The model under review builds one solid part; all positions refer to its coordinate system, in mm. A direction names the side the tool comes from. Give positions to 0.01 mm unless a question says otherwise; leave off trailing zeros. Write each loop counter-clockwise with the first axis right and the second up, starting at its lowest first coordinate (ties: lowest second). Pieces come first, ordered by that corner, then holes. Notation, with made-up numbers: M 6.25,-4.75 L 39.25,-4.75 A26 ccw 39.25,9.25 Z; hole C 43,-4 d5. An arc over 180 degrees is marked long. Write each question's results on one line, items separated by ' | '. Start each with the question number.
Autodesk Inventor part; units mm, degrees
ref_plane "YZ Plane" through (0, 0, 0) normal (1, 0, 0) x (0, 1, 0)
ref_plane "XZ Plane" through (0, 0, 0) normal (0, 1, 0) x (-1, 0, 0)
ref_plane "XY Plane" through (0, 0, 0) normal (0, 0, 1) x (1, 0, 0)
sketch "Sketch1" plane through (0, 0, 0) normal (0, 1, 0) x (-1, 0, 0)
  line L0 (17.75, -20.2435) -> (17.75, -42.6397) construction
  line L1 (13.2323, -33.7) -> (6.4845, -33.7) construction
  line L2 (35.5, -64.4) -> (35.5, -3)
  line L3 (0, -3) -> (0, -64.4)
  line L4 (32.5, 0) -> (3, 0)
  line L5 (3, -67.4) -> (32.5, -67.4)
  line L6 (16, -20.2) -> (14.2, -20.2)
  line L7 (14.2, -20.2) -> (14.2, -13.2)
  line L8 (14.2, -13.2) -> (16, -13.2)
  line L9 (16, -13.2) -> (16, -20.2)
  line L10 (31.25, -3) -> (21.25, -3)
  line L11 (21.25, -3) -> (21.25, -6.2)
  line L12 (21.25, -6.2) -> (31.25, -6.2)
  line L13 (31.25, -6.2) -> (31.25, -3)
  line L14 (14.25, -3) -> (4.25, -3)
  line L15 (4.25, -3) -> (4.25, -6.2)
  line L16 (4.25, -6.2) -> (14.25, -6.2)
  line L17 (14.25, -6.2) -> (14.25, -3)
  line L18 (31.25, -61.2) -> (21.25, -61.2)
  line L19 (21.25, -61.2) -> (21.25, -64.4)
  line L20 (21.25, -64.4) -> (31.25, -64.4)
  line L21 (31.25, -64.4) -> (31.25, -61.2)
  line L22 (14.25, -61.2) -> (4.25, -61.2)
  line L23 (4.25, -61.2) -> (4.25, -64.4)
  line L24 (4.25, -64.4) -> (14.25, -64.4)
  line L25 (14.25, -64.4) -> (14.25, -61.2)
  line L26 (10.7, -28.7) -> (7.5, -28.7)
  line L27 (7.5, -28.7) -> (7.5, -38.7)
  line L28 (7.5, -38.7) -> (10.7, -38.7)
  line L29 (10.7, -28.7) -> (10.7, -26.2)
  line L30 (10.7, -26.2) -> (13.9, -26.2)
  line L31 (13.9, -26.2) -> (13.9, -41.2)
  line L32 (13.9, -41.2) -> (10.7, -41.2)
  line L33 (10.7, -41.2) -> (10.7, -38.7)
  arc A0 (35.5, -3) -> (32.5, 0) centre (32.5, -3) ccw
  arc A1 (32.5, -67.4) -> (35.5, -64.4) centre (32.5, -64.4) ccw
  arc A2 (0, -64.4) -> (3, -67.4) centre (3, -64.4) ccw
  arc A3 (3, 0) -> (0, -3) centre (3, -3) ccw
  line L34 (16, -47.2) -> (14.2, -47.2)
  line L35 (14.2, -47.2) -> (14.2, -54.2)
  line L36 (14.2, -54.2) -> (16, -54.2)
  line L37 (16, -54.2) -> (16, -47.2)
  point P0 (0, 0)
  dimension "d22" = 7
  dimension "d24" = 1.8
  dimension "d27" = 10
  dimension "d28" = 3.2
  dimension "d30" = 3
  dimension "d31" = 7
  dimension "d33" = 10
  dimension "d34" = 15
  dimension "d35" = 6
  dimension "d39" = 7
  dimension "d52" = 35.5
  dimension "d53" = 4.25
  dimension "d54" = 7.5
  dimension "d55" = 3.5
  dimension "d56" = 55
extrude "Extrusion1" add sketch "Sketch1" along normal blind 3
properties part number "Front_wall"
(1) Add section B-B (x = -9). State the section outline as (y, z) points.
(2) Draft analysis for pull direction Z (two halves, no side actions). For faces 1 (the flat face through (-18, 3, -33)), 2 (the flat face through (-14.25, 1, -5)), 3 (the cylindrical face through (-0.9, 1.48, -66.54)), state which applies: pulls with the +Z half, pulls with the -Z half, needs draft (parallel to the pull), parting line crosses it, or undercut.
(3) Machinability: for faces 4 (the flat face through (-9, 1, -38.7)), 5 (the cylindrical face through (-34.64, 1.48, -66.5)), which of the approach directions +Z, -Z, +X, -X, +Y, -Y give a long, thin tool a straight path to every point of the face, cutting with its end or side? Answer none if there is none.
(4) Wall thickness on L1, parallel to Z at x = -14.5, y = 2.75; L2, parallel to Z at x = -12, y = 0.5; L3, parallel to X at y = 1.3, z = -62: over which ranges is each line inside the solid? List them lowest first.
(5) Add section D-D (z = -36). State the section outline as (x, y) points.
(6) Add section A-A (z = -27). State the section outline as (x, y) points.
(7) Add section C-C (x = -5). State the section outline as (y, z) points, then the cut area to 3 significant figures.
(8) Clearance check with a flat-ended pin moving along its axis: P1, Ø1.5, axis at x = -9.5, y = 1.5, coming from the +Z side. State where the tip first meets the part, or that it passes through.
Calculated:
1) outline: M 0,-67.4 L 3,-67.4 L 3,-64.4 L 0,-64.4 Z; M 0,-61.2 L 3,-61.2 L 3,-38.7 L 0,-38.7 Z; M 0,-28.7 L 3,-28.7 L 3,-6.2 L 0,-6.2 Z; M 0,-3 L 3,-3 L 3,0 L 0,0 Z
2) face 1: needs draft | face 2: undercut | face 3: pulls with the -Z half
3) face 4: +Y, -Y | face 5: -Z, -X, +Y, -Y
4) L1: z = -67.4 to -54.2, -47.2 to -20.2, -13.2 to 0 | L2: z = -67.4 to -64.4, -61.2 to -41.2, -26.2 to -6.2, -3 to 0 | L3: x = -35.5 to -31.25, -21.25 to -14.25, -4.25 to 0
5) outline: M -35.5,0 L -13.9,0 L -13.9,3 L -35.5,3 Z; M -7.5,0 L 0,0 L 0,3 L -7.5,3 Z
6) outline: M -35.5,0 L -13.9,0 L -13.9,3 L -35.5,3 Z; M -10.7,0 L 0,0 L 0,3 L -10.7,3 Z
7) outline: M 0,-67.4 L 3,-67.4 L 3,-64.4 L 0,-64.4 Z; M 0,-61.2 L 3,-61.2 L 3,-6.2 L 0,-6.2 Z; M 0,-3 L 3,-3 L 3,0 L 0,0 Z | area: 183 mm²
8) P1: stops at z = 0
